Build history of the part. All positions in model axes, mm. Face numbers are marked on the shaded views. A direction names the side the tool comes from. Give positions to 0.01 mm unless a question says otherwise; leave off trailing zeros. Write each loop counter-clockwise with the first axis right and the second up, starting at its lowest first coordinate (ties: lowest second). Pieces come first, ordered by that corner, then holes. Notation, with made-up numbers: (63, -8.75) -> (75, -8.75) arc R28 cw to (75, 22.25) -> close; hole circle Ø9 at (63.5, 89). An arc over 180 degrees is marked (long way). Put each result on its own line as item: value. Start each with the question number.
Item 1: Drill centre lines: line 1 along Z through (x, y) = (0, 2.7); line 2 along Z through (x, y) = (0, 12.25) (3 decimals). Where is each one in solid material? Low to high.
Item 2: Flat gauge pins, fed straight in: pin 1 Ø2 at (y, z) = (5.5, -2) entering from -X; pin 2 Ø1 at (x, z) = (2, 9) entering from +Y. Where does each tip first touch, or does it go through?
Item 3: Slice it at C-C, the plane y = 10.5. List the corners of the cut face in (x, z) (3 decimals), plus the area to 3 significant figures.
Item 4: Slice it at B-B, the plane x = 0. List the corners of the cut face in (y, z) (3 decimals), plus the area to 3 significant figures.
Item 5: Slice it at A-A, the plane z = 0. List the corners of the cut face in (x, y) (3 decimals).
Item 6: Slice it at D-D, the plane z = -13. List the corners of the cut face in (x, y).
Item 7: Two-plate mould, pull along Z, no slides. Class the marked faces 1, 2 and 3: pulls with the +Z half, pulls with the -Z half, needs draft (parallel to the pull), parting line crosses it, or undercut.
Item 8: Tool access for the marked faces 4, 5 and 6: list every direction of +Z, -Z, +X, -X, +Y, -Y with a clear straight run to the whole face (end or side of a thin tool).
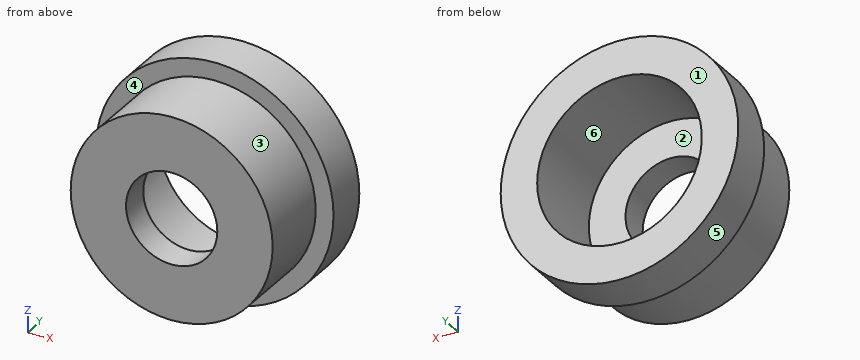
Autodesk Inventor part; units mm, degrees
ref_plane "YZ Plane" through (0, 0, 0) normal (1, 0, 0) x (0, 1, 0)
ref_plane "XZ Plane" through (0, 0, 0) normal (0, 1, 0) x (-1, 0, 0)
ref_plane "XY Plane" through (0, 0, 0) normal (0, 0, 1) x (1, 0, 0)
sketch "Sketch1" plane through (0, 0, 0) normal (0, 1, 0) x (-1, 0, 0)
  circle A0 centre (0, 0) radius 13.4938
  dimension "d0" = 26.9875
extrude "Extrusion1" add sketch "Sketch1" along normal blind 10
sketch "Sketch2" plane through (0, 10, 0) normal (0, 1, 0) x (1, 0, 0)
  circle A0 centre (0, 0) radius 13.4938
  circle A1 centre (0, 0) radius 15.875
  dimension "d3" = 31.75
extrude "Extrusion2" add sketch "Sketch2" along normal blind 6 contours A0 | A1
sketch "Sketch3" plane through (0, 16, 0) normal (0, 1, 0) x (1, 0, 0)
  circle A0 centre (0, 0) radius 11
  dimension "d6" = 22
extrude "Extrusion3" cut sketch "Sketch3" against normal blind 12
sketch "Sketch4" plane through (0, 4, 0) normal (0, 1, 0) x (1, 0, 0)
  circle A0 centre (0, 0) radius 6.1
  dimension "d9" = 12.2
extrude "Extrusion4" cut sketch "Sketch4" against normal blind 4
properties part number "Switch Cap" material "Polycarbonate, Clear"
Values follow:
1. line 1: -13.49 to -6.1, 6.1 to 13.49
1. line 2: -15.875 to -11, 11 to 15.875
2. pin 1: x = -13.46
2. pin 2: y = 4
3. outline: circle Ø31.75 at (0, 0); hole circle Ø22 at (0, 0)
3. area: 412 mm2
4. outline: (0, -13.494) -> (10, -13.494) -> (10, -15.875) -> (16, -15.875) -> (16, -11) -> (4, -11) -> (4, -6.1) -> (0, -6.1) -> close; (0, 6.1) -> (4, 6.1) -> (4, 11) -> (16, 11) -> (16, 15.875) -> (10, 15.875) -> (10, 13.494) -> (0, 13.494) -> close
4. area: 148 mm2
5. outline: (-15.875, 10) -> (-13.494, 10) -> (-13.494, 0) -> (-6.1, 0) -> (-6.1, 4) -> (-11, 4) -> (-11, 16) -> (-15.875, 16) -> close; (6.1, 0) -> (13.494, 0) -> (13.494, 10) -> (15.875, 10) -> (15.875, 16) -> (11, 16) -> (11, 4) -> (6.1, 4) -> close
6. outline: (-9.11, 10) -> (-3.62, 10) -> (-3.62, 0) -> (3.62, 0) -> (3.62, 10) -> (9.11, 10) -> (9.11, 16) -> (-9.11, 16) -> close
7. face 1: needs draft
7. face 2: undercut
7. face 3: parting line crosses it
8. face 4: -Y
8. face 5: +Y, -Y
8. face 6: +Y
